Work out the finished part from the listing and answer in its coordinate system (mm). Face numbers are marked on the shaded views. Coordinates: 2 decimals unless noted, no trailing zeros. Order: outer loops, then holes, each group sorted by start corner. A loop starts at its lowest first (then second) coordinate and runs counter-clockwise, first axis right, second up. Notation, with made-up numbers: (39.5, 28) -> (98.5, 28) arc R21 cw to (98.5, 53) -> close; hole circle Ø4 at (55, -29.75). An arc over 180 degrees is marked (long way). Write item = value, one per line. Start each with the question number.
Q1. For a pull along X with two mould halves and no side action, classify the marked faces 1 and 2 as +X half, -X half, draft (parallel to the pull), parting line (faces both ways), or undercut.
Q2. Flat-ended cylindrical pins translate along their axes: pin 1 (3 mm diameter, centred on x = -42.5, z = -12.5, fed in from +Y); pin 2 (8 mm diameter, centred on x = 22.5, y = 30, fed in from -Z); pin 3 (3 mm diameter, centred on x = 6, z = 0, fed in from -Y); pin 4 (12 mm diameter, centred on x = -8.5, y = 29, fed in from +Z). Find the tip coordinate at first contact, or state that the pin passes through.
Q3. Straight lines are drawn through the part: L1, parallel to X at y = 1.55, z = 5; L2, parallel to X at y = 31, z = -6.25; L3, parallel to Z at x = -0.5, y = 6.5. For each, find the intervals that lie inside material, in ascending order. Write a range as from..to.
Q4. The part is cut by section B-B, the plane z = -6.25. Determine the outline of the cut face in (x, y), plus the area to 3 significant figures.
Q5. The part is cut by section C-C, the plane y = 17. Determine the outline of the cut face in (x, z).
Q6. The part is cut by section A-A, the plane x = 0. Determine the outline of the cut face in (y, z).
Q7. The part is cut by section D-D, the plane x = 40. Determine the outline of the cut face in (y, z), plus the area to 3 significant figures.
Autodesk Inventor part; units mm, degrees
ref_plane "YZ Plane" through (0, 0, 0) normal (1, 0, 0) x (0, 1, 0)
ref_plane "XZ Plane" through (0, 0, 0) normal (0, 1, 0) x (-1, 0, 0)
ref_plane "XY Plane" through (0, 0, 0) normal (0, 0, 1) x (1, 0, 0)
sketch "Sketch1" plane through (0, 0, 0) normal (0, 1, 0) x (-1, 0, 0)
  line L0 (0, 0) -> (-30.6, 0)
  line L1 (0, 0) -> (30.6, 0)
  line L2 (30.6, 0) -> (41.764, -19.3366)
  line L3 (30.6, 0) -> (52.928, 0) construction
  line L4 (-30.6, 0) -> (-41.764, -19.3366)
  line L5 (-30.6, 0) -> (-8.272, 0) construction
  line L6 (0, 0) -> (0, 77)
  line L7 (0, 0) -> (0, -3)
  line L8 (-35.3569, -8.2392) -> (-32.7588, -9.7392)
  line L9 (35.0582, -7.7219) -> (32.4602, -9.2219)
  line L10 (32.4602, -9.2219) -> (28.8679, -3)
  line L11 (28.8679, -3) -> (0, -3)
  line L12 (0, -3) -> (-28.8679, -3)
  line L13 (-28.8679, -3) -> (-32.7588, -9.7392)
  line L14 (-32.7588, -9.7392) -> (-38.9714, -20.4998)
  line L15 (32.4602, -9.2219) -> (38.9714, -20.4998)
  arc A0 (38.9714, -20.4998) -> (41.764, -19.3366) centre (0, 77) ccw
  arc A1 (-41.764, -19.3366) -> (-38.9714, -20.4998) centre (0, 77) ccw
  dimension "d0" = 30.6
  dimension "d1" = 30.6
  dimension "d2" = 22.328
  dimension "d3" = 60
  dimension "d4" = 22.328
  dimension "d5" = 120
  dimension "d6" = 77
  dimension "d7" = 3
  dimension "d8" = 3
  dimension "d9" = 3
extrude "Extrusion1" add sketch "Sketch1" along normal blind 40
sketch "Sketch2" plane through (0, 0, 0) normal (0, -1, 0) x (1, 0, 0)
  line L0 (0, 0) -> (0, 5)
  circle A0 centre (0, 5) radius 1.5
  line L1 (-41.764, -19.3366) -> (-39.264, -15.0065)
  line L2 (-41.764, -19.3366) -> (-30.6, 0)
  line L3 (-39.264, -15.0065) -> (-43.5941, -12.5065)
  arc A1 (38.9714, -20.4998) -> (41.764, -19.3366) centre (0, 77) ccw
  line L4 (38.9714, -20.4998) -> (39.264, -15.0065)
  line L5 (30.6, 0) -> (41.764, -19.3366)
  line L6 (41.764, -19.3366) -> (39.264, -15.0065)
  line L7 (39.264, -15.0065) -> (43.5941, -12.5065)
  circle A2 centre (43.5941, -12.5065) radius 1.5
  circle A3 centre (-43.5941, -12.5065) radius 1.5
  circle A4 centre (-43.5941, -12.5065) radius 4
  circle A5 centre (0, 5) radius 4
  circle A6 centre (43.5941, -12.5065) radius 4
  line L8 (43.5941, -12.5065) -> (45.5941, -15.9706)
  line L9 (45.5941, -15.9706) -> (41.264, -18.4706)
  line L10 (43.5941, -12.5065) -> (41.5941, -9.0424)
  line L11 (41.5941, -9.0424) -> (37.264, -11.5424)
  line L12 (4, 5) -> (4, 0)
  line L13 (-30.6, 0) -> (30.6, 0)
  line L14 (-4, 5) -> (-4, 0)
  line L15 (-43.5941, -12.5065) -> (-45.5941, -15.9706)
  line L16 (-45.5941, -15.9706) -> (-41.264, -18.4706)
  line L17 (-41.764, -19.3366) -> (-30.6, 0)
  line L18 (-43.5941, -12.5065) -> (-41.5941, -9.0424)
  line L19 (-41.5941, -9.0424) -> (-37.264, -11.5424)
  dimension "d12" = 5
  dimension "d13" = 3
  dimension "d14" = 5
  dimension "d15" = 5
  dimension "d16" = 5.5011
  dimension "d17" = 5
  dimension "d18" = 3
  dimension "d19" = 8
  dimension "d20" = 8
  dimension "d21" = 8
extrude "Extrusion2" add sketch "Sketch2" against normal blind 3 contours L13 L14 A5 L0 | L2 L3 A4 L19 | L11 A6 L7 L5 | L0 A5 L12 L13 | A5 | L1 L16 A4 L3 | L18 A3 L15 A4 | A4 L3 A3 L18 | L7 A6 L9 L5 | L10 A2 L7 A6 | A6 L8 A2 L10 | A4 L15 A3 L3 | L18 L15 A3 | A3 L3 L18 | L7 A2 L8 A6 | L10 L7 A2 | A2 L8 L10 | A3 L15 L3 | L7 L8 A2
sketch "Sketch3" plane through (0, 3, 0) normal (0, 1, 0) x (1, 0, 0)
  arc A0 (41.5941, 9.0424) -> (45.5941, 15.9706) centre (43.5941, 12.5065) ccw
  circle A1 centre (43.5941, 12.5065) radius 1.5
  arc A2 (-45.5941, 15.9706) -> (-41.5941, 9.0424) centre (-43.5941, 12.5065) ccw
  circle A3 centre (-43.5941, 12.5065) radius 1.5
  point P0 (0, 0)
  dimension "d24" = 3
extrude "Extrusion3" cut sketch "Sketch3" against normal blind 3
properties part number "Capcture Zone"
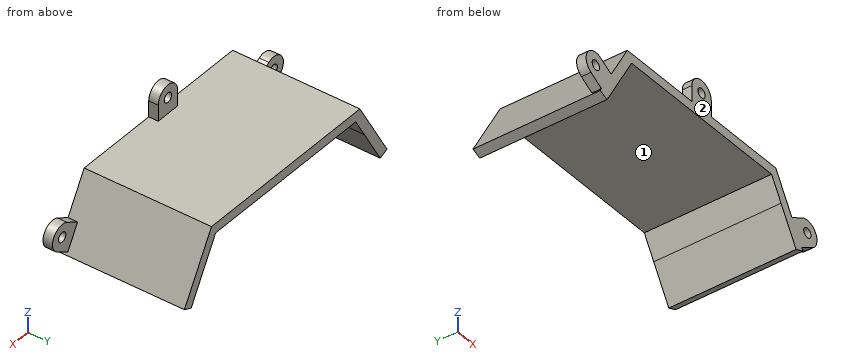
Model answer:
q1.face_1 = undercut
q1.face_2 = draft
q2.pin_1 = 3
q2.pin_2 = -3
q2.pin_3 = 0
q2.pin_4 = 0
q3.L1 = -4..-1.5, 1.5..4
q3.L2 = -34.21..-30.74, 30.74..34.21
q3.L3 = -3..0
q4.outline = (-34.21, 0) -> (-30.74, 0) -> (-30.74, 40) -> (-34.21, 40) -> close; (30.74, 0) -> (34.21, 0) -> (34.21, 40) -> (30.74, 40) -> close
q4.area = 277 mm2
q5.outline = (-41.76, -19.34) arc R104.8 ccw to (-38.97, -20.5) -> (-32.46, -9.22) -> (-28.87, -3) -> (28.87, -3) -> (32.76, -9.74) -> (38.97, -20.5) arc R105.2 ccw to (41.76, -19.34) -> (30.6, 0) -> (-30.6, 0) -> close
q6.outline = (0, -3) -> (40, -3) -> (40, 0) -> (3, 0) -> (3, 3.5) -> (0, 3.5) -> close; (0, 6.5) -> (3, 6.5) -> (3, 9) -> (0, 9) -> close
q7.outline = (0, -20.08) -> (40, -20.08) -> (40, -16.28) -> (3, -16.28) -> (3, -9.96) -> (0, -9.96) -> close
q7.area = 171 mm2
